```python
from build123d import *

# Parameters (mm, degrees)
BOSS_EXTRUDE1_DEPTH = 4


with BuildPart() as part:
    # Sketch1 → Boss-Extrude1 (new body)
    with BuildSketch(Plane.XY):
        Polygon((0, 0), (0, 90), (100, 90), (100, 2.372295937), (100, -10), (0, -10), align=None)
        with BuildLine():
            Line((7.45, 14.17243776), (7.45, -0.25030049))
            ThreePointArc((7.45, -0.25030049), (10, -2.80030049), (12.55, -0.25030049))
            Line((12.55, -0.25030049), (12.55, 14.17243776))
            ThreePointArc((12.55, 14.17243776), (10, 16.72243776), (7.45, 14.17243776))
        make_face(mode=Mode.SUBTRACT)
        with BuildLine():
            Line((87.45, 62.150571419), (87.45, 76.57330967))
            ThreePointArc((87.45, 76.57330967), (90, 79.12330967), (92.55, 76.57330967))
            Line((92.55, 76.57330967), (92.55, 62.150571419))
            ThreePointArc((92.55, 62.150571419), (90, 59.600571419), (87.45, 62.150571419))
        make_face(mode=Mode.SUBTRACT)
        with BuildLine():
            Line((92.55, 14.17243776), (92.55, -0.25030049))
            ThreePointArc((92.55, -0.25030049), (90, -2.80030049), (87.45, -0.25030049))
            Line((87.45, -0.25030049), (87.45, 14.17243776))
            ThreePointArc((87.45, 14.17243776), (90, 16.72243776), (92.55, 14.17243776))
        make_face(mode=Mode.SUBTRACT)
        with BuildLine():
            Line((12.55, 62.150571419), (12.55, 76.57330967))
            ThreePointArc((12.55, 76.57330967), (10, 79.12330967), (7.45, 76.57330967))
            Line((7.45, 76.57330967), (7.45, 62.150571419))
            ThreePointArc((7.45, 62.150571419), (10, 59.600571419), (12.55, 62.150571419))
        make_face(mode=Mode.SUBTRACT)
    extrude(amount=BOSS_EXTRUDE1_DEPTH)


solid = part.part
```
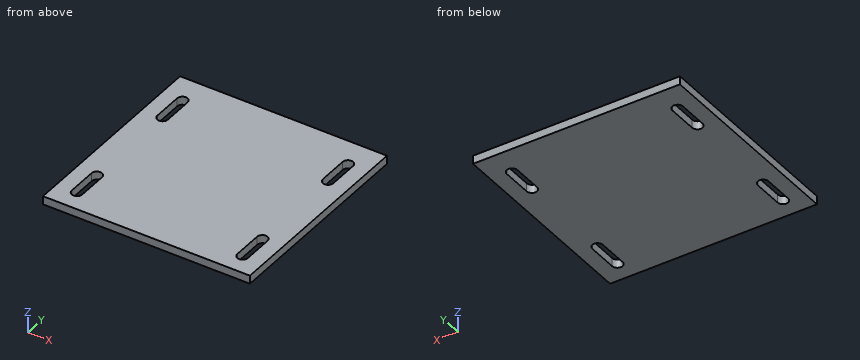
Input: part model. Units: mm. Frame: model coordinates. Give positions to 0.01 mm unless a question says otherwise; leave off trailing zeros. Order: outer loops, then holes, each group sorted by start corner. A loop starts at its lowest first (then second) coordinate and runs counter-clockwise, first axis right, second up. Notation, with made-up numbers: (51.25, -30) - (87.25, -30) arc R22 ccw to (87.25, -14) - close; hole circle Ø10 at (-18.5, -11.75). An arc over 180 degrees is marked (long way). Put each result on its own line as item: value.
Item 1: Section query A-A, the plane y = 65.5. Return loops of the section in (x, z).
Found:
outline: (0, 0) - (7.45, 0) - (7.45, 4) - (0, 4) - close; (12.55, 0) - (87.45, 0) - (87.45, 4) - (12.55, 4) - close; (92.55, 0) - (100, 0) - (100, 4) - (92.55, 4) - close
Item 2: Ray query, L1, parallel to X at y = 70.5, z = 1.5; L2, parallel to Y at x = 8, z = 0.3; L3, parallel to X at y = -2.5, z = 0.5. Return the intervals inside material, ascending. Write a range as from..to.
Found:
L1: x = 0..7.45, 12.55..87.45, 92.55..100
L2: y = -10..-1.83, 15.75..60.57, 78.16..90
L3: x = 0..8.8, 11.2..88.8, 91.2..100
Item 3: Section query C-C, the plane z = 2.15. Return loops of the section in (x, y), then the cut area to 3 significant figures.
Found:
outline: (0, -10) - (100, -10) - (100, 90) - (0, 90) - close; hole (7.45, -0.25) arc R2.55 ccw to (12.55, -0.25) - (12.55, 14.17) arc R2.55 ccw to (7.45, 14.17) - close; hole (7.45, 62.15) arc R2.55 ccw to (12.55, 62.15) - (12.55, 76.57) arc R2.55 ccw to (7.45, 76.57) - close; hole (87.45, -0.25) arc R2.55 ccw to (92.55, -0.25) - (92.55, 14.17) arc R2.55 ccw to (87.45, 14.17) - close; hole (87.45, 62.15) arc R2.55 ccw to (92.55, 62.15) - (92.55, 76.57) arc R2.55 ccw to (87.45, 76.57) - close
area: 9,620 mm^2
Item 4: Section query B-B, the plane x = 10. Return loops of the section in (y, z), then the cut area to 3 significant figures.
Found:
outline: (-10, 0) - (-2.8, 0) - (-2.8, 4) - (-10, 4) - close; (16.72, 0) - (59.6, 0) - (59.6, 4) - (16.72, 4) - close; (79.12, 0) - (90, 0) - (90, 4) - (79.12, 4) - close
area: 244 mm^2
